Design review of the part built by this model. Coordinates are the model's own, in mm. Face numbers are marked on the shaded views. A direction names the side the tool comes from. Coordinates: 2 decimals unless noted, no trailing zeros. Write each loop counter-clockwise with the first axis right and the second up, starting at its lowest first coordinate (ties: lowest second). Pieces come first, ordered by that corner, then holes. Notation, with made-up numbers: M 75.25,-21 L 96.25,-21 A22 ccw 96.25,-13 Z; hole C 1,38.5 d7. An arc over 180 degrees is marked long. One line per question, with ' | ' between items.
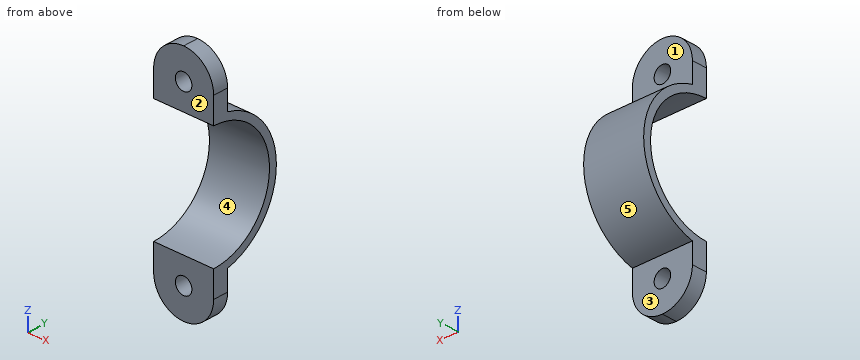
from build123d import *

# Parameters (mm, degrees)
BOSS_EXTRUDE1_DEPTH = 12
SKETCH2_R           = 1.65
CUT_EXTRUDE2_DEPTH  = 14.476258968


with BuildPart() as part:
    # Sketch1 → Boss-Extrude1 (new body)
    with BuildSketch(Plane(origin=(0, 0, 0), x_dir=(0, 0, -1), z_dir=(1, 0, 0))):
        with BuildLine():
            Line((-1.623568234, 0), (9.512622948, 0))
            ThreePointArc((9.512622948, 0), (21.512622948, 12), (33.512622948, 0))
            Line((33.512622948, 0), (44.652622948, 0))
            Line((44.652622948, 0), (44.652622948, 3))
            Line((44.652622948, 3), (34.652622948, 3))
            ThreePointArc((34.652622948, 3), (21.514527357, 13.476258968), (8.376431766, 3))
            Line((8.376431766, 3), (-1.623568234, 3))
            Line((-1.623568234, 3), (-1.623568234, 0))
        make_face()
    extrude(amount=BOSS_EXTRUDE1_DEPTH)

    # Sketch2 → Cut-Extrude2 (cut, through all)
    with BuildSketch(Plane(origin=(0, 0, 0), x_dir=(1, 0, 0), z_dir=(0, 1, 0))):
        with BuildLine():
            Line((0, 44.652622948), (0, 38.652622948))
            ThreePointArc((0, 38.652622948), (1.757359313, 42.895263636), (6, 44.652622948))
            Line((6, 44.652622948), (0, 44.652622948))
        make_face()
        with BuildLine():
            Line((12, 44.652622948), (6, 44.652622948))
            ThreePointArc((6, 44.652622948), (10.242640687, 42.895263636), (12, 38.652622948))
            Line((12, 38.652622948), (12, 44.652622948))
        make_face()
        with BuildLine():
            Line((12, -1.623568234), (12, 4.376431766))
            ThreePointArc((12, 4.376431766), (10.242640687, 0.133791079), (6, -1.623568234))
            Line((6, -1.623568234), (12, -1.623568234))
        make_face()
        with BuildLine():
            Line((0, -1.623568234), (6, -1.623568234))
            ThreePointArc((6, -1.623568234), (1.757359313, 0.133791079), (0, 4.376431766))
            Line((0, 4.376431766), (0, -1.623568234))
        make_face()
        with Locations((6, 4.376431766)):
            Circle(SKETCH2_R)
        with Locations((6, 38.652622948)):
            Circle(SKETCH2_R)
    extrude(amount=CUT_EXTRUDE2_DEPTH, mode=Mode.SUBTRACT)


solid = part.part
1. Insertion check: pin 1 Ø1 at (x, z) = (7.5, -38.5) entering from +Y; pin 2 Ø5 at (x, y) = (9, 8.5) entering from -Z; pin 3 Ø5 at (x, z) = (2, -29) entering from -Y. Each pin has a flat end and moves straight along its axis. Give the tip position at first contact, or say it passes through.
Answer sheet:
pin 1: y = 3 | pin 2: z = -33.58 | pin 3: y = 6.65
2. Take a section at D-D (x = 9.25). Write out the cut boundary in (y, z), then the cut area to 3 significant figures.
Answer sheet:
outline: M 0,-43.7 L 3,-43.7 L 3,-34.65 A13.48 ccw 3,-8.38 L 3,0.67 L 0,0.67 L 0,-9.51 A12 cw 0,-33.51 Z | area: 112 mm^2
3. Tool access review of the marked faces 1 and 2: name each direction out of +Z, -Z, +X, -X, +Y, -Y from which nothing blocks a thin tool from reaching the whole face with its end or side.
Answer sheet:
face 1: +Z, +X, -X, +Y | face 2: +Z, -Z, +X, -X, -Y
4. To check wall thickness, follow line 1 along Z through (x, y) = (6, 1.25); line 2 along Z through (x, y) = (6.75, 2.25); line 3 along Y through (x, z) = (4.5, -35). State the ranges of each line that lie inside material, in increasing order. Write a range as [from, to].
Answer sheet:
line 1: [-44.65, -40.3], [-37, -33.45], [-9.58, -6.03], [-2.73, 1.62] | line 2: [-44.61, -40.12], [-37.18, -33.3], [-9.73, -5.85], [-2.91, 1.58] | line 3: [0, 3]
5. Draft analysis for pull direction Z (two halves, no side actions). For the marked faces 3, 4 and 5, state which applies: pulls with the +Z half, pulls with the -Z half, needs draft (parallel to the pull), parting line crosses it, or undercut.
Answer sheet:
face 3: needs draft | face 4: undercut | face 5: parting line crosses it
6. Take a section at A-A (y = 7). Write out the cut boundary in (x, z).
Answer sheet:
outline: M 0,-33.03 L 12,-33.03 L 12,-31.26 L 0,-31.26 Z; M 0,-11.77 L 12,-11.77 L 12,-10 L 0,-10 Z
7. Take a section at B-B (x = 6.5). Write out the cut boundary in (y, z), then the cut area to 3 significant figures.
Answer sheet:
outline: M 0,-44.63 L 3,-44.63 L 3,-40.23 L 0,-40.23 Z; M 0,-37.08 L 3,-37.08 L 3,-34.65 A13.48 ccw 3,-8.38 L 3,-5.95 L 0,-5.95 L 0,-9.51 A12 cw 0,-33.51 Z; M 0,-2.8 L 3,-2.8 L 3,1.6 L 0,1.6 Z | area: 98.7 mm^2
8. Take a section at C-C (z = -37.5). Write out the cut boundary in (x, y).
Answer sheet:
outline: M 0,0 L 4.82,0 L 4.82,3 L 0,3 Z; M 7.18,0 L 12,0 L 12,3 L 7.18,3 Z
